```python
from build123d import *

# Parameters (mm, degrees)
SKETCH1_R                = 8
BOSS_EXTRUDE1_DEPTH      = 3
BOSS_EXTRUDE2_DEPTH      = 3
FILLET1_R                = 0.25
CIRPATTERN1_COUNT        = 11
FILLET1_OF_CIRPATTERN1_R = 0.25


with BuildPart() as part:
    # Sketch1 → Boss-Extrude1 (new body)
    with BuildSketch(Plane.XY):
        Circle(SKETCH1_R)
        with BuildLine():
            ThreePointArc((1.75, -2.436698586), (0, -3), (-1.75, -2.436698586))
            Line((-1.75, -2.436698586), (-1.75, 2.436698586))
            ThreePointArc((-1.75, 2.436698586), (0, 3), (1.75, 2.436698586))
            Line((1.75, 2.436698586), (1.75, -2.436698586))
        make_face(mode=Mode.SUBTRACT)
    extrude(amount=BOSS_EXTRUDE1_DEPTH)

    # Sketch2 → Boss-Extrude2 (add)
    with BuildSketch(Plane.XY):
        Polygon((-1.323267478, 7.75), (-1.323267478, 8.55), (-0.625, 11.25), (0.625, 11.25), (1.323267478, 8.55), (1.323267478, 7.75), align=None)
    boss_extrude2 = extrude(amount=BOSS_EXTRUDE2_DEPTH)

    # Fillet1
    fillet1_edges = [part.edges().sort_by_distance(p)[0] for p in [
        (0.625, 11.25, 1.5),
        (-0.625, 11.25, 1.5),
    ]]
    fillet(fillet1_edges, radius=FILLET1_R)

    # CirPattern1: Boss-Extrude2 ×11 about axis
    cirpattern1_axis = Axis((0, 0, 0), (0, 0, 1))
    for i in range(1, CIRPATTERN1_COUNT):
        add(boss_extrude2.rotate(cirpattern1_axis, i * 360 / CIRPATTERN1_COUNT))

    # Fillet1 of CirPattern1
    fillet1_of_cirpattern1_edges = [part.edges().sort_by_distance(p)[0] for p in [
        (-5.556425738, 9.802002755, 1.5),
        (-6.607992654, 9.126201733, 1.5),
        (-9.973725565, 5.241938893, 1.5),
        (-10.492994331, 4.104898899, 1.5),
        (-11.224437995, -0.982403529, 1.5),
        (-11.046544447, -2.219680332, 1.5),
        (-8.91147067, -6.894839773, 1.5),
        (-8.092894753, -7.839526741, 1.5),
        (-3.769174373, -10.618213105, 1.5),
        (-2.569808156, -10.970378801, 1.5),
        (2.569808156, -10.970378801, 1.5),
        (3.769174373, -10.618213105, 1.5),
        (8.092894753, -7.839526741, 1.5),
        (8.91147067, -6.894839773, 1.5),
        (11.046544447, -2.219680332, 1.5),
        (11.224437995, -0.982403529, 1.5),
        (10.492994331, 4.104898899, 1.5),
        (9.973725565, 5.241938893, 1.5),
        (6.607992654, 9.126201733, 1.5),
        (5.556425738, 9.802002755, 1.5),
    ]]
    fillet(fillet1_of_cirpattern1_edges, radius=FILLET1_OF_CIRPATTERN1_R)


solid = part.part
```
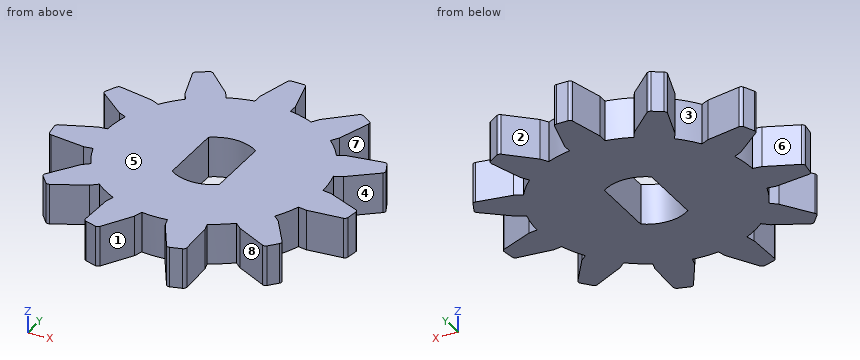
Geometry: final body of the model. Coordinates: model frame, mm. Face numbers are marked on the shaded views. A direction names the side the tool comes from. Give positions to 0.01 mm unless a question says otherwise; leave off trailing zeros. Loops run counter-clockwise (first coordinate to the right, second up) from the corner with the lowest first, then second, coordinate; pieces in that order, holes last. Notation, with made-up numbers: (-6.75, 87.25) -> (40.25, 87.25) arc R9 ccw to (40.25, 101.25) -> close; hole circle Ø8 at (54.25, 86.25). An arc over 180 degrees is marked (long way). Return JSON: item names as keys, results as strings.
Item 1: Pin query (flat end, axial travel): P1, Ø1.5, axis at x = -4.5, z = 1, coming from the +Y side; P2, Ø1.5, axis at y = 1, z = 2, coming from the +X side. Return the tip coordinate at first contact, or that it passes through.
Filled in:
{"P1": "y = 9.52", "P2": "x = 8"}
Item 2: Section A-A, the plane y = 0.75. Output: boundary loops of the cut face in (x, z).
Filled in:
{"outline": "(-7.96, 0) -> (-1.75, 0) -> (-1.75, 3) -> (-7.96, 3) -> close; (1.75, 0) -> (7.96, 0) -> (7.96, 3) -> (1.75, 3) -> close"}
Item 3: Access query for the marked faces 1, 2, 3, 4 and 5. Directions: +Z, -Z, +X, -X, +Y, -Y. A direction counts if a zero-diameter tool reaches every point of the face in a straight line with its end or side. Return the directions, or none.
Filled in:
{"face 1": "+Z, -Z, -Y", "face 2": "+Z, -Z, +Y", "face 3": "+Z, -Z", "face 4": "+Z, -Z, +X", "face 5": "+Z, +X, -X, +Y, -Y"}
Item 4: Mould query, pull axis X, two halves, no side actions, for the marked faces 6, 7 and 8. Classes: released by +X, released by -X, zero draft, split by the parting line, or undercut.
Filled in:
{"face 6": "released by -X", "face 7": "released by +X", "face 8": "undercut"}
Item 5: Line query: line 1 (X direction, y = 8, z = 0.65); line 2 (X direction, y = -7.25, z = 2.7); line 3 (X direction, y = -1.25, z = 0.3). Output: solid intervals per line, ascending.
Filled in:
{"line 1": "-6.24 to -3.61, -1.32 to 1.32, 3.61 to 6.24", "line 2": "-8.6 to -6.91, -3.51 to 3.51, 6.91 to 8.6", "line 3": "-11.19 to -1.75, 1.75 to 11.19"}
Item 6: Section B-B, the plane y = -5.25. Output: boundary loops of the cut face in (x, z), plus the area to 3 significant figures.
Filled in:
{"outline": "(-7.78, 0) -> (7.78, 0) -> (7.78, 3) -> (-7.78, 3) -> close", "area": "46.7 mm^2"}
Item 7: Section C-C, the plane x = -4.75. Output: boundary loops of the cut face in (y, z).
Filled in:
{"outline": "(-6.44, 0) -> (9.06, 0) -> (9.06, 3) -> (-6.44, 3) -> close"}
